from build123d import *

# Parameters (mm, degrees)
SKETCH1_R           = 375
BOSS_EXTRUDE1_DEPTH = 150
SKETCH2_R           = 50
CUT_EXTRUDE1_DEPTH  = 75
SCALE1_SCALE        = 0.75


with BuildPart() as part:
    # Sketch1 → Boss-Extrude1 (new body)
    with BuildSketch(Plane(origin=(0, 0, 0), x_dir=(1, 0, 0), z_dir=(0, 1, 0))):
        with Locations(Location((0, 0, 0), (0, 0, 270))):
            Circle(SKETCH1_R)
    extrude(amount=BOSS_EXTRUDE1_DEPTH)

    # Sketch2 → Cut-Extrude1 (cut)
    with BuildSketch(Plane(origin=(0, 150, 0), x_dir=(1, 0, 0), z_dir=(0, 1, 0))):
        with Locations(Location((0, 0, 0), (0, 0, 270))):
            Circle(SKETCH2_R)
    extrude(amount=-CUT_EXTRUDE1_DEPTH, mode=Mode.SUBTRACT)


with BuildPart() as part_1:
    # Scale1: scaled about (0, 74.66367713, 0)
    add(part.part.scale(SCALE1_SCALE).moved(Location((0, 18.665919282, 0))))


solid = part_1.part
Design review of the part built by this model. Coordinates are the model's own, in mm. A direction names the side the tool comes from. Give positions to 0.01 mm unless a question says otherwise; leave off trailing zeros. Write each loop counter-clockwise with the first axis right and the second up, starting at its lowest first coordinate (ties: lowest second). Pieces come first, ordered by that corner, then holes. Notation, with made-up numbers: M 53.5,32 L 66.5,32 A25 cw 66.5,44 Z; hole C 48,54 d5. An arc over 180 degrees is marked long. Return JSON: item names as keys, results as strings. Group by question number.
Item 1: Wall thickness on line 1 along X through (y, z) = (95, 0); line 2 along X through (y, z) = (104.5, -21.5); line 3 along Z through (x, y) = (-253, 74): over which ranges is each line inside the solid? List them lowest first.
Item 2: The part is to be moulded in two halves that separate along Z. For faces 3 (the flat face through (4, 131.166, 59)), 4 (the cylindrical face through (84.48, 74.128, 268.262)), 5 (the cylindrical face through (-22.818, 103.435, -29.759)), say which applies: pulls with the +Z half, pulls with the -Z half, needs draft (parallel to the pull), parting line crosses it, or undercut.
Item 3: Take a section at C-C (y = 115). Give the boundary of the cut face in (x, z), plus the area to 3 significant figures.
Item 4: Take a section at B-B (x = 0). Give the boundary of the cut face in (y, z).
Item 5: Tool access review of faces 1 (the flat face through (4, 18.666, -4)), 2 (the flat face through (1, 74.916, -1)): name each direction out of +Z, -Z, +X, -X, +Y, -Y from which nothing blocks a thin tool from reaching the whole face with its end or side.
Item 6: Take a section at A-A (z = 0). Give the boundary of the cut face in (x, y), plus the area to 3 significant figures.
Item 7: Clearance check with flat-ended pins moving along their axes: pin 1 Ø1.5 at (x, y) = (105, 59.5) entering from +Z; pin 2 Ø5 at (x, y) = (-201.5, 103.5) entering from +Z; pin 3 Ø3 at (y, z) = (94, 36.5) entering from +X. State where each tip first meets the part, or that it passes through.
Item 8: Take a section at D-D (y = 64). Give the boundary of the cut face in (x, z).
Return value:
{
 "1": {"line 1": "x = -281.25 to -37.5, 37.5 to 281.25", "line 2": "x = -280.43 to -30.72, 30.72 to 280.43", "line 3": "z = -122.85 to 122.85"},
 "2": {"face 3": "needs draft", "face 4": "parting line crosses it", "face 5": "undercut"},
 "3": {"outline": "C 0,0 d562.5; hole C 0,0 d75", "area": "244,000 mm2"},
 "4": {"outline": "M 18.67,-281.25 L 131.17,-281.25 L 131.17,-37.5 L 74.92,-37.5 L 74.92,37.5 L 131.17,37.5 L 131.17,281.25 L 18.67,281.25 Z"},
 "5": {"face 1": "+Z, -Z, +X, -X, -Y", "face 2": "+Y"},
 "6": {"outline": "M -281.25,18.67 L 281.25,18.67 L 281.25,131.17 L 37.5,131.17 L 37.5,74.92 L -37.5,74.92 L -37.5,131.17 L -281.25,131.17 Z", "area": "59,100 mm2"},
 "7": {"pin 1": "stops at z = 261.22", "pin 2": "stops at z = 198.75", "pin 3": "stops at x = 279.06"},
 "8": {"outline": "C 0,0 d562.5"}
}
